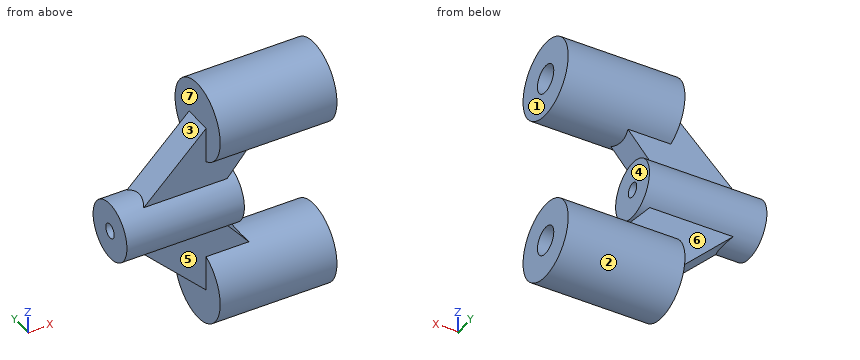
from build123d import *

# Parameters (mm, degrees)
F0_R      = 4
F1_DEPTH  = 2
F2_R      = 4
F2_R_2    = 1.45
F3_DEPTH  = 10
F5_DEPTH  = 1.5
F8_R      = 3
F9_DEPTH  = 12.07
F10_R     = 0.75
F11_DEPTH = 25


with BuildPart() as f1:
    # F0 (on Right) → F1 (new body)
    with BuildSketch(Plane.YZ):
        Circle(F0_R)
    extrude(amount=F1_DEPTH)

    # F2 (on face) → F3 (join)
    with BuildSketch(Plane.YZ.offset(2)):
        Circle(F2_R)
        Circle(F2_R_2, mode=Mode.SUBTRACT)
    extrude(amount=F3_DEPTH)

    # F4 (on Front) → F5 (join, symmetric)
    with BuildSketch(Plane.XZ):
        Polygon((0, -3), (0, 0), (-9, -9), (0, -9), (5, -3), align=None)
    extrude(amount=F5_DEPTH, both=True)

    # F8 (on plane+point) → F9 (join)
    with BuildSketch(Plane.YZ.offset(-9)):
        with Locations((0, -9)):
            Circle(F8_R)
    extrude(amount=F9_DEPTH)

    # F10 (on face) → F11 (cut)
    with BuildSketch(Plane(origin=(-9, 0, 0), x_dir=(0, -1, 0), z_dir=(-1, 0, 0))):
        with Locations((0, -9)):
            Circle(F10_R)
    extrude(amount=-F11_DEPTH, mode=Mode.SUBTRACT)

    # F13: F1 across plane


with BuildPart() as f1_1:
    add(f1.part)
    add(f1.part.mirror(Plane.XY.offset(-9)))


solid = f1_1.part
The model under review builds one solid part; all positions refer to its coordinate system, in mm. Face numbers are marked on the shaded views. A direction names the side the tool comes from. Coordinates: 2 decimals unless noted, no trailing zeros. Loops run counter-clockwise (first coordinate to the right, second up) from the corner with the lowest first, then second, coordinate; pieces in that order, holes last.
(1) Consider section A-A, the plane z = -9. Give the boundary of the cut face in (x, y), plus the area to 3 significant figures.
Determined:
outline: (-9, -3) - (3.07, -3) - (3.07, -0.75) - (-9, -0.75) - close; (-9, 0.75) - (3.07, 0.75) - (3.07, 3) - (-9, 3) - close
area: 54.3 mm2
(2) Consider section D-D, the plane y = -2.25. Give the boundary of the cut face in (x, z).
Determined:
outline: (-9, -10.98) - (3.07, -10.98) - (3.07, -7.02) - (-9, -7.02) - close; (0, -21.31) - (12, -21.31) - (12, -14.69) - (0, -14.69) - close; (0, -3.31) - (12, -3.31) - (12, 3.31) - (0, 3.31) - close
(3) Wall thickness on L1, parallel to Z at x = 4.5, y = 0; L2, parallel to Z at x = 10.75, y = -1; L3, parallel to Y at x = 5.25, z = -18: over which ranges is each line inside the solid? List them lowest first.
Determined:
L1: z = -22 to -19.45, -16.55 to -14, -4 to -1.45, 1.45 to 4
L2: z = -21.87 to -19.05, -16.95 to -14.13, -3.87 to -1.05, 1.05 to 3.87
L3: y = -4 to -1.45, 1.45 to 4
(4) Draft analysis for pull direction Z (two halves, no side actions). For the marked faces 1, 2 and 3, state which applies: +Z half, -Z half, draft (parallel to the pull), parting line (faces both ways), or undercut.
Determined:
face 1: draft
face 2: undercut
face 3: +Z half
(5) Consider section B-B, the plane x = -5.5. Give the boundary of the cut face in (y, z).
Determined:
outline: (-1.5, -12.5) - (1.5, -12.5) - (1.5, -11.6) arc R3 ccw to (1.5, -6.4) - (1.5, -5.5) - (-1.5, -5.5) - (-1.5, -6.4) arc R3 ccw to (-1.5, -11.6) - close; hole circle Ø1.5 at (0, -9)
(6) Insertion check: P1, Ø0.9, axis at y = 0, z = 0, coming from the +X side; P2, Ø1.5, axis at x = -3.5, z = -1.5, coming from the +Y side; P3, Ø12, axis at x = 8, z = -12.5, coming from the -Y side; P4, Ø2.5, axis at y = 0, z = -18, coming from the -X side. Each pin has a flat end and moves straight along its axis. Give the tip position at first contact, or say it passes through.
Determined:
P1: stops at x = 2
P2: passes through
P3: stops at y = -4
P4: stops at x = -1.25
(7) Tool access review of the marked faces 4, 5, 6 and 7: name each direction out of +Z, -Z, +X, -X, +Y, -Y from which nothing blocks a thin tool from reaching the whole face with its end or side.
Determined:
face 4: +X, +Y, -Y
face 5: -X, -Y
face 6: -X, +Y
face 7: +Z, -X
